```python
from build123d import *

# Parameters (mm, degrees)
SKETCH1_W           = 85
SKETCH1_H           = 85
BOSS_EXTRUDE1_DEPTH = 3
SKETCH5_W           = 29.5
SKETCH5_H           = 59
CUT_EXTRUDE2_DEPTH  = 4
DIAMETERHOLE2_D     = 7
FILLET2_R           = 3


with BuildPart() as part:
    # Sketch1 → Boss-Extrude1 (new body)
    with BuildSketch(Plane(origin=(0, 0, 0), x_dir=(0, 0, -1), z_dir=(1, 0, 0))):
        with Locations((42.5, 42.5)):
            Rectangle(SKETCH1_W, SKETCH1_H)
    extrude(amount=BOSS_EXTRUDE1_DEPTH)

    # Sketch5 → Cut-Extrude2 (cut, through all)
    with BuildSketch(Plane(origin=(0, 0, 0), x_dir=(0, 0, -1), z_dir=(1, 0, 0))):
        with Locations((14.75, 55.5)):
            Rectangle(SKETCH5_W, SKETCH5_H)
        with Locations((70.25, 55.5)):
            Rectangle(SKETCH5_W, SKETCH5_H)
    extrude(amount=CUT_EXTRUDE2_DEPTH, mode=Mode.SUBTRACT)

    # DiameterHole2 (through all)
    with Locations(Plane(origin=(3, 0, 0), x_dir=(0, 0, -1), z_dir=(1, 0, 0))):
        with Locations((42.5, 74), (42.5, 44), (11, 13), (73, 13)):
            Hole(DIAMETERHOLE2_D / 2)

    # Fillet2
    fillet2_edges = [part.edges().sort_by_distance(p)[0] for p in [
        (1.5, 26, 0),
        (1.5, 85, -29.5),
        (1.5, 26, -85),
        (1.5, 85, -55.5),
        (1.5, 0, -85),
        (1.5, 0, 0),
    ]]
    fillet(fillet2_edges, radius=FILLET2_R)


solid = part.part
```
Verification items for the finished model (mm, model axes). A direction names the side the tool comes from. Coordinates: 2 decimals unless noted, no trailing zeros. Loops run counter-clockwise (first coordinate to the right, second up) from the corner with the lowest first, then second, coordinate; pieces in that order, holes last. Notation, with made-up numbers: (-34, 45.5) -> (-28, 45.5) arc R35 cw to (-28, 84.5) -> close; hole circle Ø5 at (68.5, 58). An arc over 180 degrees is marked (long way). Answer in a Markdown table with one row per item. Add a question column.
1. Section check A-A, the plane y = 44. Enter the section's corners in (x, z).
2. Draft check along Z on faces 1 (the face through (1.479, 46.365, -45.08)), 2 (the face through (1, 54, -55.5)), 3 (the face through (1, 26, -69)). Enter one of: +Z half, -Z half, draft (parallel to the pull), parting line (faces both ways), or undercut.
3. Section check B-B, the plane z = -42.5. Enter the section's corners in (x, y).
4. Section check C-C, the plane y = 13. Enter the section's corners in (x, z).
5. Access from +Z, -Z, +X, -X, +Y, -Y to the whole of each face (thin tool, end or side, straight path). Record for faces 4 (the face through (1, 54, -29.5)), 5 (the face through (1.52, 84.14, -54.6)).
6. Depth check by flat-ended pin: P1, Ø0.9, axis at x = 2, y = 61, coming from the +Z side; P2, Ø11, axis at y = 44, z = -42.5, coming from the -X side; P3, Ø0.9, axis at x = 2, y = 60, coming from the -Z side; P4, Ø1.5, axis at x = 1.5, z = -15, coming from the +Y side. Enter the tip coordinate at first touch or a pass-through.
7. Section check D-D, the plane x = 0.8. Enter the section's corners in (y, z), then the cut area to 3 significant figures.
8. Material ranges on probe 1 along Y at (x, z) = (1.5, -42.5); probe 2 along Y at (x, z) = (2.2, -11); probe 3 along Y at (x, z) = (0.75, -77), recorded low to high. Write a range as [from, to].
Derived:
| question | item | result |
|---|---|---|
| 1 | outline | (0, -55.5) -> (3, -55.5) -> (3, -46) -> (0, -46) -> close; (0, -39) -> (3, -39) -> (3, -29.5) -> (0, -29.5) -> close |
| 2 | face 1 | undercut |
| 2 | face 2 | -Z half |
| 2 | face 3 | draft |
| 3 | outline | (0, 0) -> (3, 0) -> (3, 40.5) -> (0, 40.5) -> close; (0, 47.5) -> (3, 47.5) -> (3, 70.5) -> (0, 70.5) -> close; (0, 77.5) -> (3, 77.5) -> (3, 85) -> (0, 85) -> close |
| 4 | outline | (0, -85) -> (3, -85) -> (3, -76.5) -> (0, -76.5) -> close; (0, -69.5) -> (3, -69.5) -> (3, -14.5) -> (0, -14.5) -> close; (0, -7.5) -> (3, -7.5) -> (3, 0) -> (0, 0) -> close |
| 5 | face 4 | +Z, +X, -X, +Y |
| 5 | face 5 | -Z, +X, -X, +Y |
| 6 | P1 | stops at z = -29.5 |
| 6 | P2 | stops at x = 0 |
| 6 | P3 | stops at z = -55.5 |
| 6 | P4 | stops at y = 26 |
| 7 | outline | (0, -82) arc R3 ccw to (3, -85) -> (23, -85) arc R3 ccw to (26, -82) -> (26, -55.5) -> (82, -55.5) arc R3 ccw to (85, -52.5) -> (85, -32.5) arc R3 ccw to (82, -29.5) -> (26, -29.5) -> (26, -3) arc R3 ccw to (23, 0) -> (3, 0) arc R3 ccw to (0, -3) -> close; hole circle Ø7 at (13, -73); hole circle Ø7 at (13, -11); hole circle Ø7 at (44, -42.5); hole circle Ø7 at (74, -42.5) |
| 7 | area | 3,580 mm² |
| 8 | probe 1 | y = [0, 40.5], [47.5, 70.5], [77.5, 85] |
| 8 | probe 2 | y = [0, 9.5], [16.5, 26] |
| 8 | probe 3 | y = [0, 26] |
